```python
from build123d import *

# Parameters (mm, degrees)
SKETCH1_R           = 9
BOSS_EXTRUDE1_DEPTH = 12.5
SKETCH2_R           = 2.5
CUT_EXTRUDE1_DEPTH  = 29.053520278
SKETCH3_R           = 1.5
CUT_EXTRUDE2_DEPTH  = 18.839562775
SKETCH4_R           = 1.5
CUT_EXTRUDE3_DEPTH  = 18.839562946


with BuildPart() as part:
    # Sketch1 → Boss-Extrude1 (new, symmetric)
    with BuildSketch(Plane.XY):
        Circle(SKETCH1_R)
    extrude(amount=BOSS_EXTRUDE1_DEPTH, both=True)

    # Sketch2 → Cut-Extrude1 (cut, through all)
    with BuildSketch(Plane.XY.offset(12.5)):
        Circle(SKETCH2_R)
    extrude(amount=-CUT_EXTRUDE1_DEPTH, mode=Mode.SUBTRACT)

    # Sketch3 → Cut-Extrude2 (cut, through all)
    with BuildSketch(Plane(origin=(0, 0, 0), x_dir=(1, 0, 0), z_dir=(0, 1, 0))):
        with Locations(Location((0, 10, 0), (0, 0, 90))):
            Circle(SKETCH3_R)
        with Locations(Location((0, -10, 0), (0, 0, 90))):
            Circle(SKETCH3_R)
    extrude(amount=CUT_EXTRUDE2_DEPTH, mode=Mode.SUBTRACT)

    # Sketch4 → Cut-Extrude3 (cut, through all)
    with BuildSketch(Plane(origin=(0, 0, 0), x_dir=(0, 0, -1), z_dir=(1, 0, 0))):
        with Locations(Location((-10, 0, 0), (0, 0, 180))):
            Circle(SKETCH4_R)
        with Locations(Location((10, 0, 0), (0, 0, 180))):
            Circle(SKETCH4_R)
    extrude(amount=CUT_EXTRUDE3_DEPTH, mode=Mode.SUBTRACT)


solid = part.part
```
Could you check a few things on this model? Use its own coordinates, in mm. A direction names the side the tool comes from. Give positions to 0.01 mm unless a question says otherwise; leave off trailing zeros. Loops run counter-clockwise (first coordinate to the right, second up) from the corner with the lowest first, then second, coordinate; pieces in that order, holes last. Notation, with made-up numbers: (-2.5, 42) -> (4.5, 42) arc R22 cw to (4.5, 58) -> close; hole circle Ø11 at (0, 76.5). An arc over 180 degrees is marked (long way). Put each result on its own line as item: value.
(1) For faces 5 (the face through (5.45, -0.07, 8.5)), 6 (the face through (2, -2, -12.5)), 7 (the face through (-0.07, 5.45, -8.5)), which set-ups out of +Z, -Z, +X, -X, +Y, -Y let a thin tool reach every point of the face, with its end or its side?
Computed:
face 5: +X
face 6: -Z, +X, -X, +Y, -Y
face 7: +Y
(2) Imagine slicing it at A-A on z = -11. Write out the boundary of the cut face in (x, y).
Computed:
outline: (-1.12, 2.24) -> (-1.12, 8.93) arc R9 ccw (long way) to (8.93, -1.12) -> (2.24, -1.12) arc R2.5 cw (long way) to start; (1.12, 2.24) arc R2.5 cw to (2.24, 1.12) -> (8.93, 1.12) arc R9 ccw to (1.12, 8.93) -> close
(3) Please list where these lines run through material, in increasing order: probe 1 along Z at (x, y) = (-1.25, 4); probe 2 along X at (y, z) = (4.5, 10); probe 3 along Y at (x, z) = (1.5, 0.75). Write a range as [from, to].
Computed:
probe 1: [-12.5, -10.83], [-9.17, 9.17], [10.83, 12.5]
probe 2: [-7.79, -1.5], [1.5, 7.79]
probe 3: [-8.87, -2], [2, 8.87]
(4) I'm going to push flat-ended pins straight in: pin 1 Ø1.5 at (x, z) = (5, -9.5) entering from -Y; pin 2 Ø5 at (x, z) = (6.5, 1) entering from -Y; pin 3 Ø3 at (x, y) = (0, 0) entering from +Z; pin 4 Ø1 at (x, z) = (6.5, 3.5) entering from -Y. Where does each tip first touch, or does it pass through?
Computed:
pin 1: y = -7.93
pin 2: y = -8.06
pin 3: through
pin 4: y = -6.71
(5) Imagine slicing it at B-B on y = 0.5. Write out the boundary of the cut face in (x, z), plus the area to 3 significant figures.
Computed:
outline: (-8.99, -12.5) -> (-2.45, -12.5) -> (-2.45, 12.5) -> (-8.99, 12.5) -> close; (2.45, -12.5) -> (8.99, -12.5) -> (8.99, -11.41) -> (2.45, -11.41) -> close; (2.45, -8.59) -> (8.99, -8.59) -> (8.99, 8.59) -> (2.45, 8.59) -> close; (2.45, 11.41) -> (8.99, 11.41) -> (8.99, 12.5) -> (2.45, 12.5) -> close
area: 290 mm^2
(6) Thinking about a two-plate mould opening in X: for faces 1 (the face through (-1.951, -8.786, 0.175)), 2 (the face through (-2, -1.5, 0.2)), 3 (the face through (5.45, -0.07, -11.5)), 4 (the face through (-0.07, 5.45, 11.5)), which applies, pulls with the +X half, pulls with the -X half, needs draft (parallel to the pull), parting line crosses it, or undercut?
Computed:
face 1: parting line crosses it
face 2: undercut
face 3: needs draft
face 4: undercut
(7) Imagine slicing it at D-D on z = 2.75. Write out the boundary of the cut face in (x, y).
Computed:
outline: circle Ø18 at (0, 0); hole circle Ø5 at (0, 0)
